Verification items for this drawing (mm, ordinates from the low corner). Give positions to 0.01 mm unless a question says otherwise; leave off trailing zeros. Order: outer loops, then holes, each group sorted by start corner. A loop starts at its lowest first (then second) coordinate and runs counter-clockwise, first axis right, second up.
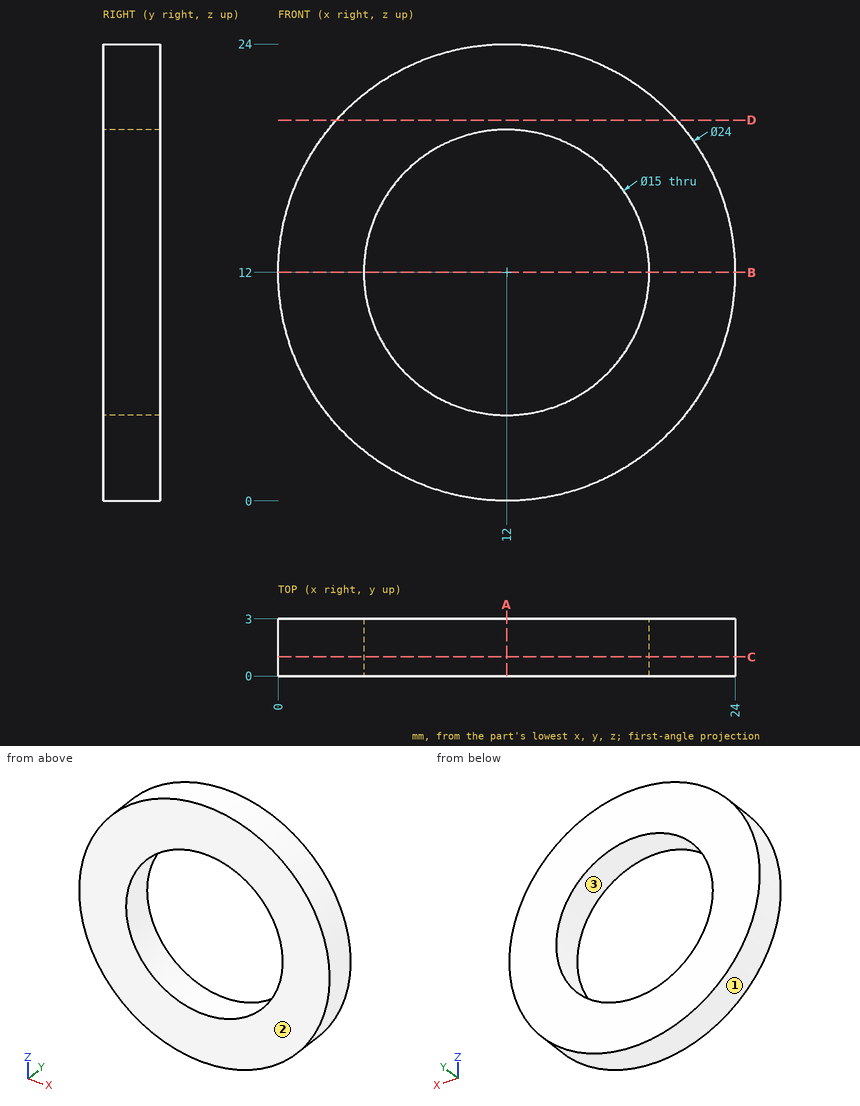
Q1. Release check for a two-part mould opening along X. For the marked faces 1, 2 and 3 record: pulls with the +X half, pulls with the -X half, needs draft (parallel to the pull), parting line crosses it, or undercut.
Q2. Gauge pin test, flat ends, axial feed: P1, Ø1, axis at x = 15, z = 7, coming from the +Y side; P2, Ø1.5, axis at y = 2.5, z = 15, coming from the -X side. Record the tip position at first contact, or that the pin passes through.
Q3. Cross-section at B-B, the plane z = 12. Record the boundary of the cut face in (x, y), and give its area (3 significant figures).
Q4. Thickness scan on L1, parallel to Z at x = 12, y = 1.05; L2, parallel to Z at x = 16.5, y = 2.4; L3, parallel to X at y = 1.55, z = 13. Record the ranges inside material, lowest first.
Q5. Cross-section at A-A, the plane x = 12. Record the boundary of the cut face in (y, z), and give its area (3 significant figures).
Q6. Cross-section at C-C, the plane y = 1. Record the boundary of the cut face in (x, z), and give its area (3 significant figures).
Q7. Cross-section at D-D, the plane z = 20. Record the boundary of the cut face in (x, y).
Answers follow:
1. face 1: parting line crosses it
1. face 2: needs draft
1. face 3: undercut
2. P1: passes through
2. P2: stops at x = 0.21
3. outline: (0, 0) - (4.5, 0) - (4.5, 3) - (0, 3) - close; (19.5, 0) - (24, 0) - (24, 3) - (19.5, 3) - close
3. area: 27.0 mm2
4. L1: z = 0 to 4.5, 19.5 to 24
4. L2: z = 0.88 to 6, 18 to 23.12
4. L3: x = 0.04 to 4.57, 19.43 to 23.96
5. outline: (0, 0) - (3, 0) - (3, 4.5) - (0, 4.5) - close; (0, 19.5) - (3, 19.5) - (3, 24) - (0, 24) - close
5. area: 27.0 mm2
6. outline: circle Ø24 at (12, 12); hole circle Ø15 at (12, 12)
6. area: 276 mm2
7. outline: (3.06, 0) - (20.94, 0) - (20.94, 3) - (3.06, 3) - close
